Design review of the part shown in the three views and the two pictorial views. Dimensions are in mm from the part's minimum x, y and z. A direction names the side the tool comes from. Coordinates: 2 decimals unless noted, no trailing zeros. Write each loop counter-clockwise with the first axis right and the second up, starting at its lowest first coordinate (ties: lowest second). Pieces come first, ordered by that corner, then holes. Notation, with made-up numbers: M 28.5,56 L 69.5,56 A34 cw 69.5,87 Z; hole C 56.5,-14 d7. An arc over 180 degrees is marked long. Answer as a JSON object with one key per item and string values.
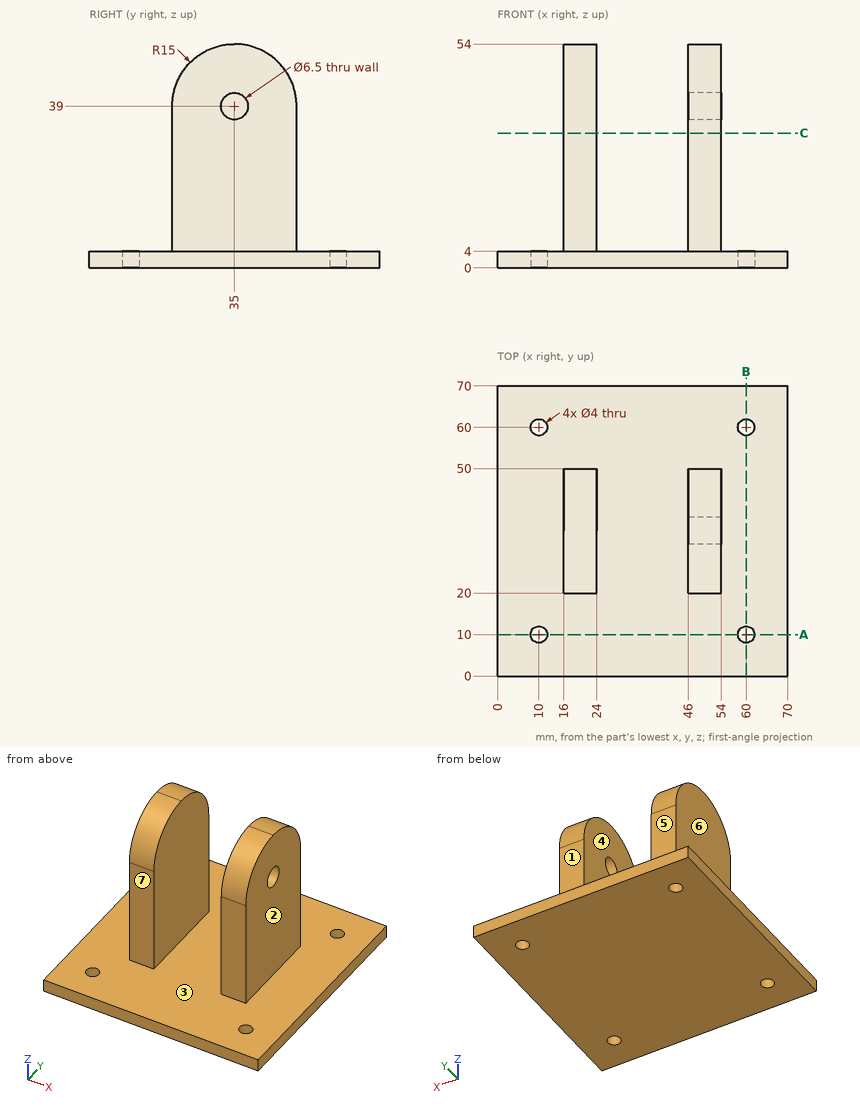
(1) Wall thickness on line 1 along Y through (x, z) = (10, 1.15); line 2 along X through (y, z) = (33, 11); line 3 along Z through (x, y) = (59, 30.5): over which ranges is each line inside the solid? List them lowest first. Write a range as from..to.
Results list:
{"line 1": "0..8, 12..58, 62..70", "line 2": "16..24, 46..54", "line 3": "0..4"}
(2) For the marked faces 4, 5, 6 and 7, list the 3-axis set-ups (+Z, -Z, +X, -X, +Y, -Y) from which the entire face can be reached by the end or side of a thin tool; tool diameter is ignored.
Results list:
{"face 4": "+Z, +Y, -Y", "face 5": "+Z, +X, -X, +Y", "face 6": "+Z, -X, +Y, -Y", "face 7": "+Z, +X, -X, -Y"}
(3) For pin 1 Ø24 at (y, z) = (36.5, 25.5) entering from -X; pin 2 Ø10 at (x, z) = (47.5, 31) entering from +Y; pin 3 Ø1.5 at (y, z) = (42.5, 15.5) entering from +X, all flat-tipped, find the tip position at first contact; note any pin that passes through.
Results list:
{"pin 1": "x = 16", "pin 2": "y = 50", "pin 3": "x = 54"}
(4) Draft analysis for pull direction X (two halves, no side actions). For the marked faces 1, 2 and 3, state which applies: released by +X, released by -X, zero draft, split by the parting line, or undercut.
Results list:
{"face 1": "zero draft", "face 2": "released by +X", "face 3": "undercut"}
(5) Add section C-C on z = 32.5. Give the boundary of the cut face in (x, y), and give its area (3 significant figures).
Results list:
{"outline": "M 16,20 L 24,20 L 24,50 L 16,50 Z; M 46,20 L 54,20 L 54,50 L 46,50 Z", "area": "480 mm²"}
(6) Add section A-A on y = 10. Give the boundary of the cut face in (x, z), and give its area (3 significant figures).
Results list:
{"outline": "M 0,0 L 8,0 L 8,4 L 0,4 Z; M 12,0 L 58,0 L 58,4 L 12,4 Z; M 62,0 L 70,0 L 70,4 L 62,4 Z", "area": "248 mm²"}
